from build123d import *

# Parameters (mm, degrees)
F0_W      = 81.28
F0_H      = 147.32
F1_DEPTH  = 10.16
F2_W      = 77.216
F2_H      = 143.256
F3_DEPTH  = 8.89
F5_DEPTH  = 10.16
F6_W      = 31.75
F6_H      = 8.255
F7_DEPTH  = 3.302
F8_W      = 29.21
F8_H      = 6.985
F9_DEPTH  = 2.159
F11_DEPTH = 25.4
F13_DEPTH = 5.08


with BuildPart() as f1:
    # F0 (on Front) → F1 (new body)
    with BuildSketch(Plane.XZ):
        with Locations((-6.703687, 25.66678)):
            Rectangle(F0_W, F0_H)
    extrude(amount=F1_DEPTH)

    # F2 (on face) → F3 (cut)
    with BuildSketch(Plane.XZ.offset(10.16)):
        with Locations((-6.703687, 25.66678)):
            Rectangle(F2_W, F2_H)
    extrude(amount=-F3_DEPTH, mode=Mode.SUBTRACT)

    # F4 (on face) → F5 (join)
    with BuildSketch(Plane.XZ.offset(10.16)):
        with BuildLine():
            ThreePointArc((-45.311687, 92.21478), (-41.719585, 93.702678), (-40.231687, 97.29478))
            Line((-40.231687, 97.29478), (-45.311687, 97.29478))
            Line((-45.311687, 97.29478), (-45.311687, 92.21478))
        make_face()
        with BuildLine():
            Line((31.904313, 97.29478), (26.824313, 97.29478))
            ThreePointArc((26.824313, 97.29478), (28.31221, 93.702678), (31.904313, 92.21478))
            Line((31.904313, 92.21478), (31.904313, 97.29478))
        make_face()
        with BuildLine():
            ThreePointArc((-40.231687, -45.96122), (-41.719585, -42.369117), (-45.311687, -40.88122))
            Line((-45.311687, -40.88122), (-45.311687, -45.96122))
            Line((-45.311687, -45.96122), (-40.231687, -45.96122))
        make_face()
        with BuildLine():
            ThreePointArc((31.904313, -40.88122), (28.31221, -42.369117), (26.824313, -45.96122))
            Line((26.824313, -45.96122), (31.904313, -45.96122))
            Line((31.904313, -45.96122), (31.904313, -40.88122))
        make_face()
    extrude(amount=-F5_DEPTH)

    # F6 (on face) → F7 (join)
    with BuildSketch(Plane.XY.offset(99.32678)):
        with Locations((-6.703687, -6.0325)):
            Rectangle(F6_W, F6_H)
    extrude(amount=F7_DEPTH)

    # F8 (on face) → F9 (cut)
    with BuildSketch(Plane.XY.offset(102.62878)):
        with Locations((-6.703687, -6.6675)):
            Rectangle(F8_W, F8_H)
    extrude(amount=-F9_DEPTH, mode=Mode.SUBTRACT)

    # F10 (on face) → F11 (cut)
    with BuildSketch(Plane.XY.offset(100.46978)):
        with BuildLine():
            Line((-14.3501, -10.16), (0.942725, -10.16))
            ThreePointArc((0.942725, -10.16), (-6.703687, -6.985), (-14.3501, -10.16))
        make_face()
    extrude(amount=-F11_DEPTH, mode=Mode.SUBTRACT)

    # F12 (on face) → F13 (cut)
    with BuildSketch(Plane(origin=(0, 0, 0), x_dir=(-1, 0, 0), z_dir=(0, 1, 0))):
        with BuildLine():
            ThreePointArc((-31.968985, 92.467752), (-28.556487, 93.881254), (-27.142985, 97.293752))
            Line((-27.142985, 97.293752), (-27.142985, 99.32678))
            Line((-27.142985, 99.32678), (-33.936313, 99.32678))
            Line((-33.936313, 99.32678), (-33.936313, 92.467752))
            Line((-33.936313, 92.467752), (-31.968985, 92.467752))
        make_face()
        with BuildLine():
            Line((40.479984, 99.32678), (40.479984, 97.294772))
            ThreePointArc((40.479984, 97.294772), (41.893487, 93.882275), (45.305984, 92.468772))
            Line((45.305984, 92.468772), (47.343687, 92.468772))
            Line((47.343687, 92.468772), (47.343687, 99.32678))
            Line((47.343687, 99.32678), (40.479984, 99.32678))
        make_face()
        with BuildLine():
            ThreePointArc((-27.082259, -45.961216), (-28.495762, -42.548718), (-31.908259, -41.135216))
            Line((-31.908259, -41.135216), (-33.936313, -41.135216))
            Line((-33.936313, -41.135216), (-33.936313, -47.99322))
            Line((-33.936313, -47.99322), (-27.082259, -47.99322))
            Line((-27.082259, -47.99322), (-27.082259, -45.961216))
        make_face()
        with BuildLine():
            Line((47.343687, -41.20655), (45.310436, -41.20655))
            ThreePointArc((45.310436, -41.20655), (41.897938, -42.620053), (40.484436, -46.03255))
            Line((40.484436, -46.03255), (40.484436, -47.99322))
            Line((40.484436, -47.99322), (47.343687, -47.99322))
            Line((47.343687, -47.99322), (47.343687, -41.20655))
        make_face()
    extrude(amount=-F13_DEPTH, mode=Mode.SUBTRACT)


solid = f1.part
Can you work these out from the model? Positions are in its coordinate system, mm. A direction names the side the tool comes from. Coordinates: 2 decimals unless noted, no trailing zeros. Write each loop counter-clockwise with the first axis right and the second up, starting at its lowest first coordinate (ties: lowest second). Pieces come first, ordered by that corner, then holes. Notation, with made-up numbers: (-3.75, -7) - (31.25, -7) arc R31 ccw to (31.25, 20) - close; hole circle Ø10 at (45.5, 38.5). An arc over 180 degrees is marked (long way). Return JSON: item names as keys, results as strings. Group by question number.
Item 1: If we section it at A-A (z = 1.5): Write out the boundary of the cut face in (x, y), then the cut area to 3 significant figures.
Item 2: Please list where these lines run through material, in increasing order: probe 1 along X at (y, z) = (-6.75, 22); probe 2 along Z at (x, y) = (-7.5, -3.75); probe 3 along Z at (x, y) = (-1, -1.5).
Item 3: I'm going to push flat-ended pins straight in: pin 1 Ø1.7 at (y, z) = (-8, 101.5) entering from -X; pin 2 Ø2.5 at (y, z) = (-7, 101) entering from +X; pin 3 Ø3.5 at (y, z) = (-5.5, 101) entering from -X; pin 4 Ø5 at (x, y) = (-2.5, -7.5) entering from +Z. Where does each tip first touch, or does it pass through?
Item 4: If we section it at B-B (x = 18.5): Write out the boundary of the cut face in (y, z), then the cut area to 3 significant figures.
Item 5: We'd pull the mould along X, two halves only. Please class faces 6 (the face through (31, -5.08, 96)), 7 (the face through (28.273, -5.777, 93.742)), 8 (the face through (-41.856, -2.504, 93.92)): pulls with the +X half, pulls with the -X half, needs draft (parallel to the pull), parting line crosses it, or undercut.
Item 6: Which directions (+Z, -Z, +X, -X, +Y, -Y) give clear straight access to the entire face, cutting with the end or side of a thin tool? Please do faces 1 (the face through (32.2, -10.16, 33.2)), 2 (the face through (28.35, -5.78, -42.33)), 3 (the face through (31, -5.08, -45)), 4 (the face through (-22.579, -6, 101)), 5 (the face through (28.594, -2.504, 93.844)).
Return value:
{
 "1": {"outline": "(-47.34, -10.16) - (-45.31, -10.16) - (-45.31, -1.27) - (31.9, -1.27) - (31.9, -10.16) - (33.94, -10.16) - (33.94, 0) - (-47.34, 0) - close", "area": "139 mm^2"},
 "2": {"probe 1": "x = -47.34 to -45.31, 31.9 to 33.94", "probe 2": "z = -47.99 to -45.96, 97.29 to 100.47", "probe 3": "z = -47.99 to -45.96, 97.29 to 99.33"},
 "3": {"pin 1": "stops at x = -22.58", "pin 2": "stops at x = 9.17", "pin 3": "stops at x = -47.34", "pin 4": "stops at z = 100.47"},
 "4": {"outline": "(-10.16, -47.99) - (0, -47.99) - (0, 99.33) - (-10.16, 99.33) - (-10.16, 97.29) - (-1.27, 97.29) - (-1.27, -45.96) - (-10.16, -45.96) - close", "area": "223 mm^2"},
 "5": {"face 6": "needs draft", "face 7": "undercut", "face 8": "pulls with the -X half"},
 "6": {"face 1": "+Z, -Z, +X, -X, -Y", "face 2": "-Y", "face 3": "-Z, +X, +Y", "face 4": "+Z, -X, +Y, -Y", "face 5": "+Z, +X, +Y"}
}
